Answer from the drawing. Dimensions are ordinates in mm from the lowest x, y and z of the part. Give positions to 0.01 mm unless a question says otherwise; leave off trailing zeros. Write each loop counter-clockwise with the first axis right and the second up, starting at its lowest first coordinate (ties: lowest second). Pieces come first, ordered by that corner, then holes.
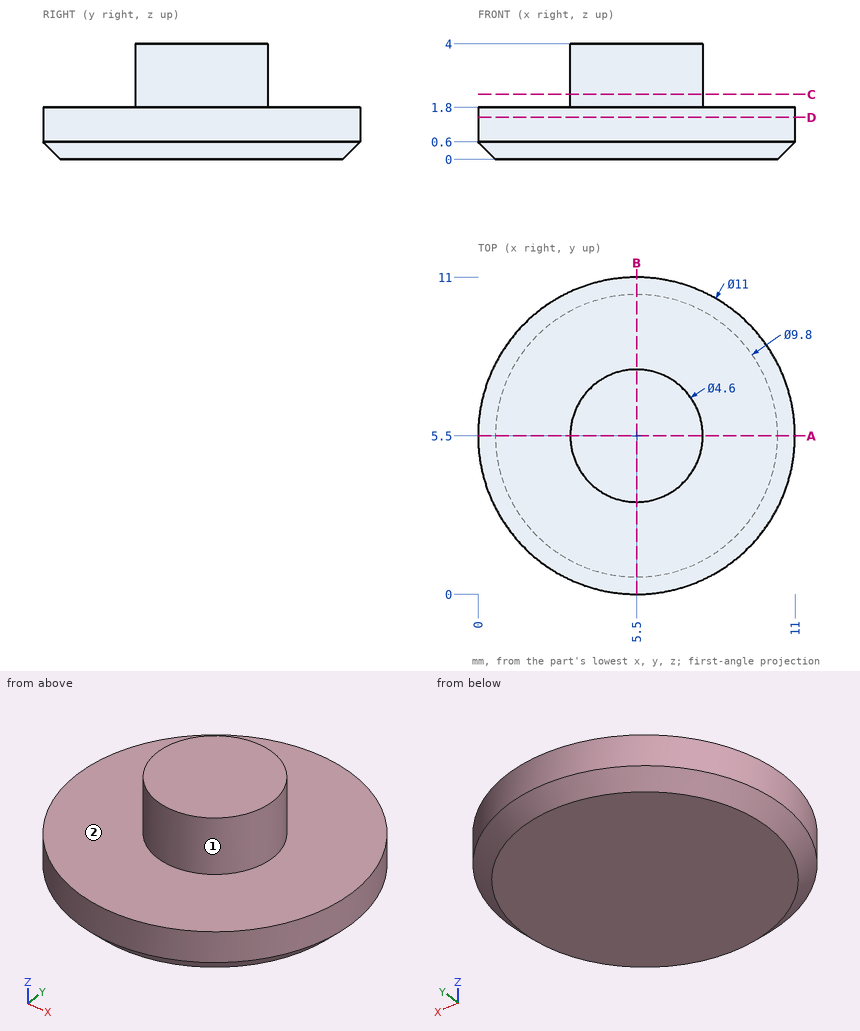
Item 1: This flat-tipped pin is pushed along its axis until it touches: P1, Ø1.5, axis at y = 2.5, z = 2, coming from the -X side. Where does it stop, or does it pass through?
Conclusion:
P1: stops at x = 0.49
Item 2: Determine the mould class of the marked faces 1 and 2 for opening direction Y: pulls with the +Y half, pulls with the -Y half, needs draft (parallel to the pull), parting line crosses it, or undercut.
Conclusion:
face 1: parting line crosses it
face 2: needs draft
Item 3: A cutting plane is placed at A-A, the plane y = 5.5. Give the vertices of the cut face in (x, z), plus the area to 3 significant figures.
Conclusion:
outline: (0, 0.6) - (0.6, 0) - (10.4, 0) - (11, 0.6) - (11, 1.8) - (7.8, 1.8) - (7.8, 4) - (3.2, 4) - (3.2, 1.8) - (0, 1.8) - close
area: 29.6 mm2
Item 4: A cutting plane is placed at C-C, the plane z = 2.25. Give the vertices of the cut face in (x, y).
Conclusion:
outline: circle Ø4.6 at (5.5, 5.5)
Item 5: Consider probe 1 along Z at (x, y) = (2.5, 6.25); probe 2 along X at (y, z) = (3.5, 2.15); probe 3 along X at (y, z) = (5.75, 2.4). Determine where each line is inside the solid, lowest interval first.
Conclusion:
probe 1: z = 0 to 1.8
probe 2: x = 4.36 to 6.64
probe 3: x = 3.21 to 7.79
Item 6: A cutting plane is placed at D-D, the plane z = 1.45. Give the vertices of the cut face in (x, y).
Conclusion:
outline: circle Ø11 at (5.5, 5.5)
